The listing builds one solid part. Answer for the finished solid, in the listing's coordinates (mm). Give positions to 0.01 mm unless a question says otherwise; leave off trailing zeros. Write each loop counter-clockwise with the first axis right and the second up, starting at its lowest first coordinate (ties: lowest second). Pieces come first, ordered by that corner, then holes. Notation, with made-up numbers: (22.5, -28) - (76.5, -28) arc R13 cw to (76.5, -19) - close; hole circle Ø11 at (77.5, -24). An arc over 180 degrees is marked (long way). Return JSON: item names as keys, results as strings.
from build123d import *

# Parameters (mm, degrees)
F0_W     = 27.6
F0_H     = 0.15
F0_H_2   = 0.9
F1_DEPTH = 13.8
F2_DEPTH = 15.9
F3_DEPTH = 7.15
F4_DEPTH = 6.25


with BuildPart() as f1:
    # F0 (on Right) → F1 (new body, symmetric)
    with BuildSketch(Plane.YZ):
        with Locations((-13.8, 0.975)):
            Rectangle(F0_W, F0_H)
        with Locations((-13.8, 0.45)):
            Rectangle(F0_W, F0_H_2)
    extrude(amount=F1_DEPTH, both=True)

    # F0 (on Right) → F2 (join, symmetric)
    with BuildSketch(Plane.YZ):
        Polygon((-35.1, 0.9), (-35.1, 0), (-35.1, -0.1), (2.2, -0.1), (2.2, 0.9), (0, 0.9), (0, 0), (-27.6, 0), (-27.6, 0.9), align=None)
        with Locations((-13.8, 0.45)):
            Rectangle(F0_W, F0_H_2)
    extrude(amount=F2_DEPTH, both=True)

    # F0 (on Right) → F3 (join, symmetric)
    with BuildSketch(Plane.YZ):
        with BuildLine():
            Line((-35.1, -0.1), (-35.1, 0))
            Line((-35.1, 0), (-39.1, 0))
            ThreePointArc((-39.1, 0), (-39.75, -0.65), (-39.1, -1.3))
            Line((-39.1, -1.3), (-38.1, -1.3))
            Line((-38.1, -1.3), (-38.1, -1.2))
            Line((-38.1, -1.2), (-39.1, -1.2))
            ThreePointArc((-39.1, -1.2), (-39.65, -0.65), (-39.1, -0.1))
            Line((-39.1, -0.1), (-35.1, -0.1))
        make_face()
    extrude(amount=F3_DEPTH, both=True)

    # F0 (on Right) → F4 (join, symmetric)
    with BuildSketch(Plane.YZ):
        Polygon((-38.1, -1.2), (-38.1, -1.3), (-37.1, -1.3), (-37.1, -1.5), (-31.1, -1.5), (-31.1, -1.3), (-31.1, -1.2), align=None)
    extrude(amount=F4_DEPTH, both=True)


solid = f1.part
Item 1: A cutting plane is placed at C-C on z = -0.65. Determine the outline of the cut face in (x, y).
Answer below:
{"outline": "(-7.15, -39.75) - (7.15, -39.75) - (7.15, -39.65) - (-7.15, -39.65) - close"}
Item 2: Flat-ended cylindrical pins translate along their axes: P1, Ø2, axis at x = -6.5, y = -34, coming from the +Z side; P2, Ø2, axis at x = 12, y = -26, coming from the -Z side; P3, Ø1.2, axis at x = -3, y = -36.5, coming from the +Z side; P4, Ø1.5, axis at x = 12.5, z = -1, coming from the -Y side. Find the tip coordinate at first contact, or state that the pin passes through.
Answer below:
{"P1": "stops at z = 0.9", "P2": "stops at z = -0.1", "P3": "stops at z = 0", "P4": "passes through"}
Item 3: A cutting plane is placed at B-B on x = -10.5. Determine the outline of the cut face in (y, z).
Answer below:
{"outline": "(-35.1, -0.1) - (2.2, -0.1) - (2.2, 0.9) - (0, 0.9) - (0, 1.05) - (-27.6, 1.05) - (-27.6, 0.9) - (-35.1, 0.9) - close"}
Item 4: A cutting plane is placed at D-D on y = -30.5. Determine the outline of the cut face in (x, z).
Answer below:
{"outline": "(-15.9, -0.1) - (15.9, -0.1) - (15.9, 0.9) - (-15.9, 0.9) - close"}
Item 5: The mould has two halves that part along Z. Classify faces 1 (the face through (0, -35, -1.2)), 2 (the face through (0, -14, 1.05)), 3 (the face through (-15.9, -16.7, 0.4)), 4 (the face through (0, -34, -1.5)): +Z half, -Z half, draft (parallel to the pull), parting line (faces both ways), or undercut.
Answer below:
{"face 1": "undercut", "face 2": "+Z half", "face 3": "draft", "face 4": "-Z half"}
Item 6: Consider L1, parallel to Z at x = 7, y = -28; L2, parallel to Z at x = 9.5, y = -17; L3, parallel to Y at x = -3.5, z = 0.5. Determine where each line is inside the solid, lowest interval first.
Answer below:
{"L1": "z = -0.1 to 0.9", "L2": "z = -0.1 to 1.05", "L3": "y = -35.1 to 2.2"}
Item 7: A cutting plane is placed at A-A on y = -17. Determine the outline of the cut face in (x, z), then the cut area to 3 significant figures.
Answer below:
{"outline": "(-15.9, -0.1) - (15.9, -0.1) - (15.9, 0.9) - (13.8, 0.9) - (13.8, 1.05) - (-13.8, 1.05) - (-13.8, 0.9) - (-15.9, 0.9) - close", "area": "35.9 mm²"}
